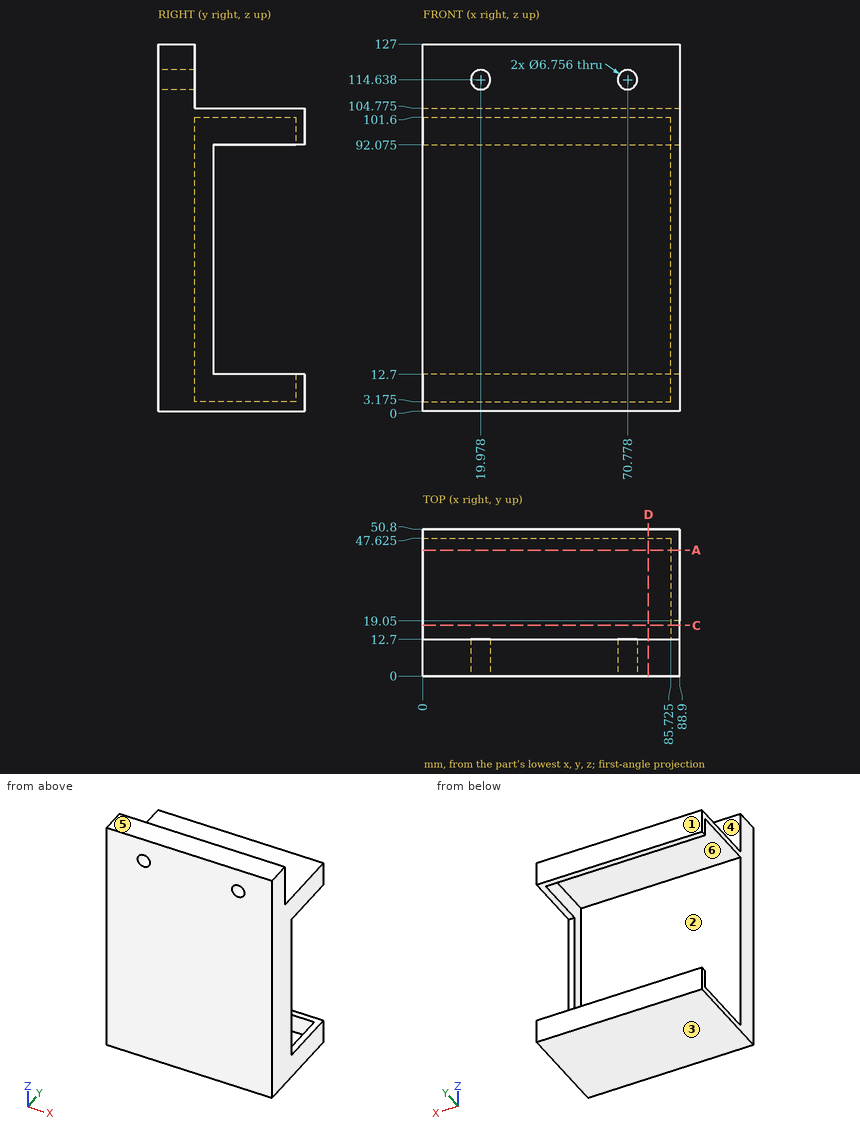
Verification items for this drawing (mm, ordinates from the low corner). A direction names the side the tool comes from. Give positions to 0.01 mm unless a question says otherwise; leave off trailing zeros. Loops run counter-clockwise (first coordinate to the right, second up) from the corner with the lowest first, then second, coordinate; pieces in that order, holes last. Notation, with made-up numbers: M -17,31 L 39,31 A28 ccw 39,69 Z; hole C 10,7.5 d4. An arc over 180 degrees is marked long. Answer in a Markdown table with one row per item.
1) Thickness scan on line 1 (Z direction, x = 14.5, y = 19.5) (1 decimal); line 2 (Y direction, x = 59, z = 12) (1 decimal); line 3 (Y direction, x = 25, z = 52). Record the ranges inside material, lowest first.
Solutions:
| item | result |
|---|---|
| line 1 | z = 0 to 3.2, 101.6 to 104.8 |
| line 2 | y = 0 to 12.7, 47.6 to 50.8 |
| line 3 | y = 0 to 12.7 |
2) Cross-section at A-A (y = 43.5). Enter the section's corners in (x, z) (1 decimal), plus the area to 3 significant figures.
Solutions:
| item | result |
|---|---|
| outline | M 0,0 L 88.9,0 L 88.9,12.7 L 85.7,12.7 L 85.7,3.2 L 0,3.2 Z; M 0,101.6 L 85.7,101.6 L 85.7,92.1 L 88.9,92.1 L 88.9,104.8 L 0,104.8 Z |
| area | 625 mm^2 |
3) Depth check by flat-ended pin: pin 1 (10.5 mm diameter, centred on x = 62, y = 35, fed in from +Z) (1 decimal); pin 2 (1 mm diameter, centred on x = 87, z = 63, fed in from +Y); pin 3 (9 mm diameter, centred on x = 70.78, z = 114.64, fed in from +Y). Enter the tip coordinate at first touch or a pass-through.
Solutions:
| item | result |
|---|---|
| pin 1 | stops at z = 104.8 |
| pin 2 | stops at y = 19.05 |
| pin 3 | stops at y = 12.7 |
4) Cross-section at D-D (x = 78). Enter the section's corners in (y, z) (1 decimal).
Solutions:
| item | result |
|---|---|
| outline | M 0,0 L 50.8,0 L 50.8,12.7 L 47.6,12.7 L 47.6,3.2 L 12.7,3.2 L 12.7,101.6 L 47.6,101.6 L 47.6,92.1 L 50.8,92.1 L 50.8,104.8 L 12.7,104.8 L 12.7,127 L 0,127 Z |
5) Tool access check on the marked faces 4, 5 and 6. Record the directions out of +Z, -Z, +X, -X, +Y, -Y that give a thin tool (end or side, any length) a straight path to the whole face; none if there is none.
Solutions:
| item | result |
|---|---|
| face 4 | +Z, +X, -X, +Y |
| face 5 | +Z, +X, -X, +Y, -Y |
| face 6 | -X |
6) Mould release check, pull along Z, two halves, no side actions. Record for the marked faces 1, 2 and 3: released by +Z, released by -Z, zero draft, split by the parting line, or undercut.
Solutions:
| item | result |
|---|---|
| face 1 | zero draft |
| face 2 | undercut |
| face 3 | released by -Z |
7) Cross-section at C-C (y = 17.5). Enter the section's corners in (x, z) (1 decimal).
Solutions:
| item | result |
|---|---|
| outline | M 0,0 L 88.9,0 L 88.9,104.8 L 0,104.8 L 0,101.6 L 85.7,101.6 L 85.7,3.2 L 0,3.2 Z |
